Design review of the part built by this model. Coordinates are the model's own, in mm. A direction names the side the tool comes from. Coordinates: 2 decimals unless noted, no trailing zeros. Loops run counter-clockwise (first coordinate to the right, second up) from the corner with the lowest first, then second, coordinate; pieces in that order, holes last. Notation, with made-up numbers: (79, 17) -> (98, 17) arc R23 ccw to (98, 55) -> close; hole circle Ø1 at (67.5, -24.5). An arc over 180 degrees is marked (long way). One line per item, written item: value. Start each with the question number.
1. Insertion check: pin 1 (2.5 mm diameter, centred on x = 38.49, y = 424.78, fed in from -Z); pin 2 (1.5 mm diameter, centred on x = 21, z = 1.5, fed in from -Y). Each pin has a flat end and moves straight along its axis. Give the tip position at first contact, or say it passes through.
2. Add section B-B on y = 408. Write out the cut boundary in (x, z), plus the area to 3 significant figures.
3. Draft analysis for pull direction Y (two halves, no side actions). For faces 1 (the flat face through (118, 421, 3)), 2 (the flat face through (178, 391, 1)), 3 (the flat face through (184.39, 376.18, 1.48)), state which applies: pulls with the +Y half, pulls with the -Y half, needs draft (parallel to the pull), parting line crosses it, or undercut.
4. Add section D-D on y = 370. Write out the cut boundary in (x, z), plus the area to 3 significant figures.
5. Machinability: for faces 4 (the flat face through (47.91, 375.86, 1.48)), 5 (the flat face through (54.127, 390.855, 1.479)), which of the approach directions +Z, -Z, +X, -X, +Y, -Y give a long, thin tool a straight path to every point of the face, cutting with its end or side? Answer none if there is none.
6. Add section A-A on x = 79. Write out the cut boundary in (y, z), plus the area to 3 significant figures.
7. Add section C-C on z = 0.7. Give the number of separate pieces and of enclosed holes in the cut face, plus the area to 3 significant figures.
8. For probe 1 along X at (y, z) = (422, 1.45); probe 2 along Y at (x, z) = (83, 2.5); probe 3 along X at (y, z) = (425, 1.65), list the stretches that pass through material, from the lowest coordinate up.
```python
from build123d import *

# Parameters (mm, degrees)
SKETCH1_R          = 1.6
EXTRUDE1_DEPTH     = 3
SKETCH2_R          = 1.6
CUT_EXTRUDE1_DEPTH = 5


with BuildPart() as part:
    # Sketch1 → Extrude1 (new body)
    with BuildSketch(Plane.XY):
        Polygon((-21.510078765, 432.284503285), (253.489921235, 432.284503285), (253.489921235, 387.497048214), (195.708175305, 387.497048214), (172.745594885, 364.534467794), (59.234247585, 364.534467794), (36.271667166, 387.497048214), (-21.510078765, 387.497048214), align=None)
        with Locations((-11.510078765, 422.284503285)):
            Circle(SKETCH1_R, mode=Mode.SUBTRACT)
        with Locations((-11.510078765, 397.497048214)):
            Circle(SKETCH1_R, mode=Mode.SUBTRACT)
        with Locations((243.489921235, 397.497048214)):
            Circle(SKETCH1_R, mode=Mode.SUBTRACT)
        with Locations((243.489921235, 422.284503285)):
            Circle(SKETCH1_R, mode=Mode.SUBTRACT)
        Polygon((-1.510078765, 417.284503285), (233.489921235, 417.284503285), (233.489921235, 402.497048214), (189.494971869, 402.497048214), (166.53239145, 379.534467794), (65.44745102, 379.534467794), (42.484870601, 402.497048214), (-1.510078765, 402.497048214), align=None, mode=Mode.SUBTRACT)
    extrude(amount=EXTRUDE1_DEPTH)

    # Sketch2 → Cut-Extrude1 (cut)
    with BuildSketch(Plane(origin=(0, 0, 0), x_dir=(-1, 0, 0), z_dir=(0, 0, -1))):
        with Locations((-38.489921235, 424.784503285)):
            Circle(SKETCH2_R)
        with Locations((-8.489921235, 424.784503285)):
            Circle(SKETCH2_R)
        with Locations((-38.489921235, 394.997048214)):
            Circle(SKETCH2_R)
        with Locations((-8.489921235, 394.997048214)):
            Circle(SKETCH2_R)
    extrude(amount=-CUT_EXTRUDE1_DEPTH, mode=Mode.SUBTRACT)


solid = part.part
```
Worked answers:
1. pin 1: passes through
1. pin 2: stops at y = 387.5
2. outline: (-21.51, 0) -> (-1.51, 0) -> (-1.51, 3) -> (-21.51, 3) -> close; (233.49, 0) -> (253.49, 0) -> (253.49, 3) -> (233.49, 3) -> close
2. area: 120 mm²
3. face 1: needs draft
3. face 2: undercut
3. face 3: pulls with the -Y half
4. outline: (53.77, 0) -> (178.21, 0) -> (178.21, 3) -> (53.77, 3) -> close
4. area: 373 mm²
5. face 4: +Z, -Z, -X, -Y
5. face 5: +Z, -Z
6. outline: (364.53, 0) -> (379.53, 0) -> (379.53, 3) -> (364.53, 3) -> close; (417.28, 0) -> (432.28, 0) -> (432.28, 3) -> (417.28, 3) -> close
6. area: 90.0 mm²
7. separate pieces: 1
7. enclosed holes: 9
7. area: 9,060 mm²
8. probe 1: x = -21.51 to -13.08, -9.94 to 241.92, 245.06 to 253.49
8. probe 2: y = 364.53 to 379.53, 417.28 to 432.28
8. probe 3: x = -21.51 to 6.9, 10.08 to 36.9, 40.08 to 253.49
